Drawing for the job (mm, zero at the part's lowest x, y, z). A direction names the side the tool comes from. Give positions to 0.01 mm unless a question says otherwise; leave off trailing zeros. Order: outer loops, then holes, each group sorted by start corner. A loop starts at its lowest first (then second) coordinate and runs counter-clockwise, first axis right, second up. Notation, with made-up numbers: (82, 25) -> (93, 25) arc R19 cw to (93, 42) -> close; hole circle Ø3 at (35, 87). An arc over 180 degrees is marked (long way). Use one line per item in the form item = value. Start each with the question number.
1) Drop flat-ended pins along their axis: P1, Ø10, axis at y = 22.5, z = 9, coming from the -X side; P2, Ø3.5, axis at x = 52, y = 11, coming from the +Z side; P3, Ø2.5, axis at x = 34.5, z = 26.5, coming from the +Y side; P4, Ø2.5, axis at x = 2.5, y = 8.35, coming from the -Z side. Give the stop position or say it passes through.
2) Tool access for the marked faces 1, 2 and 3: list every direction of +Z, -Z, +X, -X, +Y, -Y with a clear straight run to the whole face (end or side of a thin tool).
3) Cut at B-B, the plane x = 34.5. Give the cut face in (y, z).
4) Cut at C-C, the plane y = 8.35. Give the cut face in (x, z).
5) Cut at D-D, the plane z = 12.5. Give the cut face in (x, y).
6) Cut at A-A, the plane z = 19.5. Give the cut face in (x, y).
7) Probe line 1 (X direction, y = 0.6, z = 12.5); line 2 (Y direction, x = 52.5, z = 24.25); line 3 (X direction, y = 11.25, z = 22). List the from-to ranges inside material, lowest first.
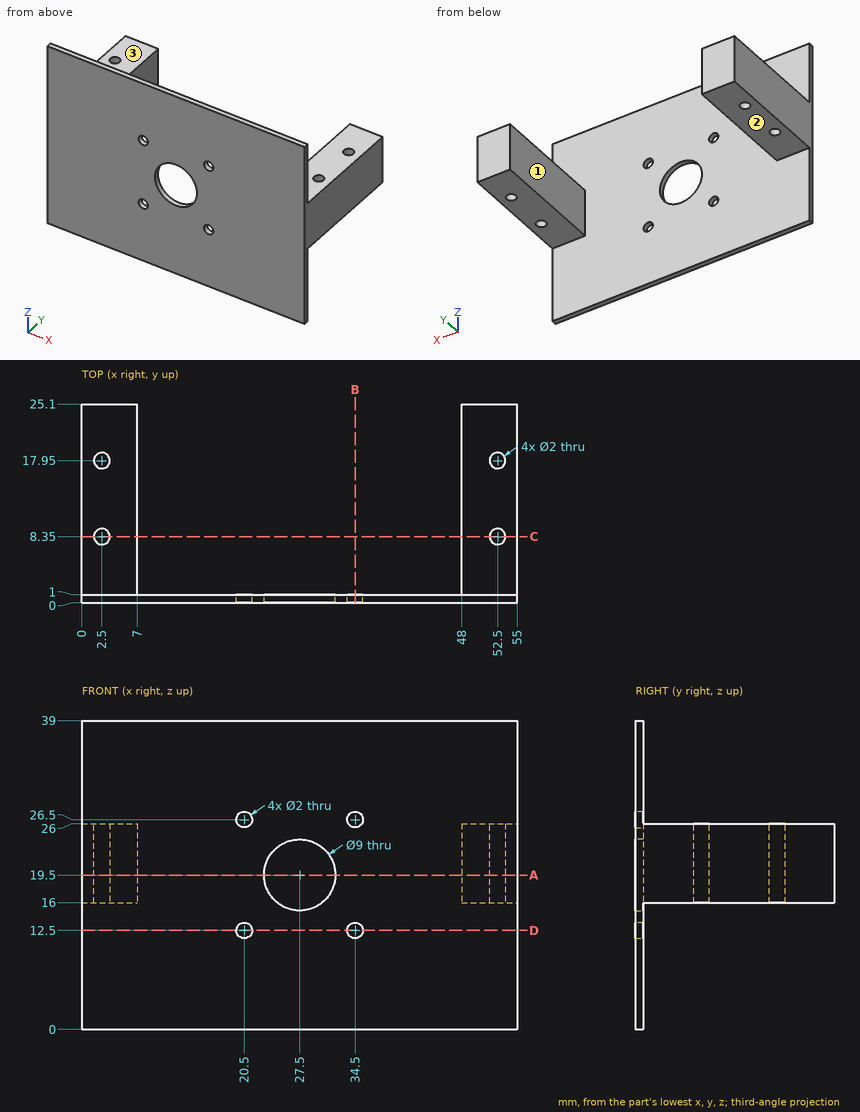
Result:
q1.P1 = through
q1.P2 = 26
q1.P3 = 1
q1.P4 = 16
q2.face_1 = +Z, -Z, +Y
q2.face_2 = -Z, +X, -X, +Y
q2.face_3 = +Z, +X, -X, +Y
q3.outline = (0, 0) -> (1, 0) -> (1, 11.5) -> (0, 11.5) -> close; (0, 13.5) -> (1, 13.5) -> (1, 25.5) -> (0, 25.5) -> close; (0, 27.5) -> (1, 27.5) -> (1, 39) -> (0, 39) -> close
q4.outline = (0, 16) -> (1.5, 16) -> (1.5, 26) -> (0, 26) -> close; (3.5, 16) -> (7, 16) -> (7, 26) -> (3.5, 26) -> close; (48, 16) -> (51.5, 16) -> (51.5, 26) -> (48, 26) -> close; (53.5, 16) -> (55, 16) -> (55, 26) -> (53.5, 26) -> close
q5.outline = (0, 0) -> (19.5, 0) -> (19.5, 1) -> (0, 1) -> close; (21.5, 0) -> (33.5, 0) -> (33.5, 1) -> (21.5, 1) -> close; (35.5, 0) -> (55, 0) -> (55, 1) -> (35.5, 1) -> close
q6.outline = (0, 0) -> (23, 0) -> (23, 1) -> (7, 1) -> (7, 25.1) -> (0, 25.1) -> close; (32, 0) -> (55, 0) -> (55, 25.1) -> (48, 25.1) -> (48, 1) -> (32, 1) -> close; hole circle Ø2 at (2.5, 8.35); hole circle Ø2 at (2.5, 17.95); hole circle Ø2 at (52.5, 8.35); hole circle Ø2 at (52.5, 17.95)
q7.line_1 = 0 to 19.5, 21.5 to 33.5, 35.5 to 55
q7.line_2 = 0 to 7.35, 9.35 to 16.95, 18.95 to 25.1
q7.line_3 = 0 to 7, 48 to 55
